Work out the finished part from the listing and answer in its coordinate system (mm). A direction names the side the tool comes from. Coordinates: 2 decimals unless noted, no trailing zeros. Order: outer loops, then holes, each group sorted by start corner. A loop starts at its lowest first (then second) coordinate and runs counter-clockwise, first axis right, second up.
1. The part is cut by section C-C, the plane z = 101.75. Give the vertices of the cut face in (x, y).
2. The part is cut by section A-A, the plane z = 10. Give the vertices of the cut face in (x, y), then the cut area to 4 significant figures.
3. The part is cut by section D-D, the plane x = 85. Give the vertices of the cut face in (y, z), then the cut area to 3 significant figures.
4. A tool of negligible diameter and unlimited length cuts with its end or side. For faces 1 (the flat face through (40, 15, 100)), 2 (the flat face through (8, 5, 16)), 3 (the flat face through (55, 10, 100)), from which of +Z, -Z, +X, -X, +Y, -Y can it reach the whole face along a straight path? Write none if from no direction.
5. The part is cut by section B-B, the plane x = 10. Give the vertices of the cut face in (y, z).
6. Find the intervals of material crossed by probe 1 along Z at (x, y) = (10, 12.75); probe 2 along Z at (x, y) = (85, 4); probe 3 along X at (y, z) = (10.5, 65), in increasing order.
7. Flat-ended cylindrical pins translate along their axes: pin 1 Ø5.5 at (x, z) = (58.25, 108.25) entering from -Y; pin 2 Ø3 at (x, z) = (20.61, 56.56) entering from +Y; pin 3 Ø3 at (y, z) = (11.5, 97) entering from -X; pin 4 Ø2 at (x, y) = (86.5, 7.5) entering from +Z. Find the tip coordinate at first contact, or state that the pin passes through.
8. Determine the mould class of faces 4 (the flat face through (0, 10, 41)), 5 (the cylindrical face through (37.54, 9.86, 5.38)), 6 (the flat face through (51, 0, 41)) for opening direction X: +X half, -X half, draft (parallel to the pull), parting line (faces both ways), or undercut.
Autodesk Inventor part; units mm, degrees
ref_plane "YZ Plane" through (0, 0, 0) normal (1, 0, 0) x (0, 1, 0)
ref_plane "XZ Plane" through (0, 0, 0) normal (0, 1, 0) x (-1, 0, 0)
ref_plane "XY Plane" through (0, 0, 0) normal (0, 0, 1) x (1, 0, 0)
sketch "Boceto1" plane through (0, 0, 0) normal (0, 1, 0) x (-1, 0, 0)
  line L0 (100, 80) -> (-100, 80)
  line L1 (-100, 80) -> (-100, -80)
  line L2 (-100, -80) -> (100, -80)
  line L3 (100, -80) -> (100, 80)
  line L4 (100, 80) -> (-100, -80) construction
  line L5 (-100, 80) -> (100, -80) construction
  point P0 (0, 0)
  dimension "d0" = 200
  dimension "d1" = 160
extrude "Extrusión1" add sketch "Boceto1" along normal blind 20
sketch "Boceto2" plane through (0, 20, 0) normal (0, 1, 0) x (1, 0, 0)
  line L0 (-100, 80) -> (-100, -80)
  line L1 (-100, 80) -> (-70, 80)
  line L2 (-70, 80) -> (-70, 40)
  line L3 (-70, 40) -> (-100, 40)
  line L4 (-100, 40) -> (-100, 80)
  line L5 (100, 80) -> (-100, 80)
  line L6 (0, 80) -> (0, 40)
  line L7 (100, 80) -> (70, 80)
  line L8 (70, 80) -> (70, 40)
  line L9 (70, 40) -> (100, 40)
  line L10 (100, 40) -> (100, 80)
  point P0 (0, 0)
  dimension "d4" = 30
  dimension "d5" = 40
extrude "Extrusión2" cut sketch "Boceto2" against normal blind 10
sketch "Boceto3" plane through (0, 20, 0) normal (0, 1, 0) x (1, 0, 0)
  line L0 (-70, 80) -> (-70, 40)
  line L1 (-70, 80.0001) -> (-70, 40)
  line L2 (-70, 40) -> (-100, 40)
  line L3 (-100, 40) -> (-100, 80.0001)
  line L4 (-100, 40) -> (-70, 40)
  line L5 (-70, 40) -> (-70, 80)
  line L6 (-70, 80) -> (-100, 80)
  line L7 (-100, 80) -> (-100, 40)
  circle A0 centre (-88.25, 58.25) radius 1.75
  circle A1 centre (-81.75, 51.75) radius 1.75
  line L8 (100, 80) -> (-100, 80)
  line L9 (0, 80) -> (0, 56.5)
  circle A2 centre (88.25, 58.25) radius 1.75
  circle A3 centre (81.75, 51.75) radius 1.75
  point P0 (0, 0)
  point P1 (-64.3507, 80)
  point P2 (-74.3507, 0)
  point P3 (-85, 80)
  dimension "d23" = 21.75
  dimension "d24" = 11.75
  dimension "d26" = 11.75
hole "Agujero1" at (-81.75, 20, -51.75) at (-88.25, 20, -58.25) at (81.75, 20, -51.75) at (88.25, 20, -58.25) direction (0, -1, 0) diameter 3.5 end through all
sketch "Boceto4" plane through (-100, 0, 80) normal (0, 0, 1) x (1, 0, 0)
  line L0 (30, 20) -> (60, 20)
  line L1 (60, 20) -> (60, 10)
  line L2 (60, 10) -> (30, 10)
  line L3 (30, 10) -> (30, 20)
  line L4 (0, 0) -> (0, 20)
  line L5 (100, 0) -> (100, 10)
  line L6 (170, 20) -> (140, 20)
  line L7 (140, 20) -> (140, 10)
  line L8 (140, 10) -> (170, 10)
  line L9 (170, 10) -> (170, 20)
  dimension "d34" = 30
  dimension "d35" = 10
  dimension "d36" = 30
extrude "Extrusión3" add sketch "Boceto4" along normal blind 40
sketch "Boceto5" plane through (0, 20, 0) normal (0, 1, 0) x (1, 0, 0)
  line L0 (59.9999, -50) -> (69.9999, -50)
  line L1 (49.9999, -101.75) -> (49.9999, -79.9497)
  line L2 (59.9999, -108.25) -> (59.9999, -50)
  line L3 (40, -80) -> (69.9999, -80)
  line L4 (49.9999, -79.9497) -> (40, -80)
  circle A0 centre (51.7499, -101.75) radius 1.75
  circle A1 centre (58.2499, -108.25) radius 1.75
  line L5 (69.9999, -80) -> (69.9999, -120)
  line L6 (40, -120) -> (40, -80)
  line L7 (69.9999, -120) -> (40, -120)
  line L8 (0, -50) -> (0, -71.75)
  line L9 (-40, -120) -> (-40, -80)
  line L10 (-49.9999, -101.75) -> (-49.9999, -79.9497)
  circle A2 centre (-51.7499, -101.75) radius 1.75
  circle A3 centre (-58.2499, -108.25) radius 1.75
  line L11 (-40, -80) -> (-69.9999, -80)
  line L12 (-69.9999, -120) -> (-40, -120)
  line L13 (-69.9999, -80) -> (-69.9999, -120)
  line L14 (-59.9999, -108.25) -> (-59.9999, -50)
  line L15 (-40, -120) -> (-69.9999, -120)
  line L16 (-69.9999, -80) -> (-69.9999, -120)
  line L17 (-40, -120) -> (-70, -120)
  line L18 (-40, -80) -> (-40, -120)
  line L19 (-59.9999, -110) -> (-49.9999, -110)
  line L20 (-49.9999, -110) -> (-49.9999, -100)
  line L21 (-49.9999, -100) -> (-59.9999, -100)
  line L22 (-59.9999, -100) -> (-59.9999, -110)
  line L23 (-100, 40) -> (-100, -80)
  point P0 (0, 0)
  point P1 (-56.75, -68.25)
  point P2 (-63.25, -61.75)
  point P3 (63.25, -61.75)
  point P4 (56.75, -68.25)
  dimension "d45" = 3.5
  dimension "d46" = 3.5
  dimension "d39" = 10
  dimension "d40" = 10
  dimension "d41" = 40
  dimension "d42" = 0
  dimension "d43" = 6.5
  dimension "d44" = 6.5
  dimension "d47" = 11.7499
  dimension "d48" = 11.75
  dimension "d49" = 0
  dimension "d50" = 11.75
  dimension "d51" = 0
  dimension "d97" = 40.0001
hole "Agujero2" at (-58.2499, 20, 108.25) at (-51.7499, 20, 101.75) at (51.7499, 20, 101.75) at (58.2499, 20, 108.25) direction (0, -1, 0) diameter 3.5 end through all
sketch "Boceto6" plane through (0, 20, 0) normal (0, 1, 0) x (1, 0, 0)
  circle A0 centre (-60.569, -13.1067) radius 10
  circle A1 centre (-29.569, -59.1067) radius 3.5
  line L0 (-60.569, -13.1067) -> (-39.0083, -13.1067)
  circle A2 centre (-29.569, 25.8933) radius 3.5
  circle A3 centre (-88.569, 25.8933) radius 3.5
  circle A4 centre (-88.569, -59.1067) radius 3.5
  line L1 (70.4544, -63.0517) -> (18.4544, -63.0517)
  line L2 (18.4544, -63.0517) -> (18.4544, 6.9483)
  line L3 (18.4544, 6.9483) -> (70.4544, 6.9483)
  line L4 (70.4544, 6.9483) -> (70.4544, -63.0517)
  line L5 (70.4544, 6.9483) -> (48.4544, 6.9483)
  line L6 (48.4544, 6.9483) -> (48.4544, 48.9483)
  line L7 (48.4544, 48.9483) -> (70.4544, 48.9483)
  line L8 (70.4544, 48.9483) -> (70.4544, 6.9483)
  line L9 (77.2288, -8.158) -> (77.2281, -5.6604)
  circle A5 centre (63.7706, -5.7606) radius 1.75
  line L10 (70.7641, -24.1464) -> (70.7641, 22.2796)
  circle A6 centre (35.8307, -5.7609) radius 1.75
  line L11 (25.1581, -13.2381) -> (25.1581, -10.7404)
  circle A7 centre (68.8507, -57.8309) radius 1.75
  line L12 (26.4277, 35.0051) -> (26.4277, 37.5029)
  circle A8 centre (20.6074, -56.5614) radius 1.75
  line L13 (18.6941, -55.9176) -> (70.7641, -55.9176)
  line L14 (18.6941, -55.9176) -> (18.6941, -7.6743)
  line L15 (44.7291, -55.9176) -> (44.7291, -31.7959)
  line L16 (63.7706, -28.0517) -> (26.4277, -28.0517)
  line L17 (44.7291, -23.5247) -> (44.7291, -31.7959)
  point P0 (0, 0)
  point P1 (-60.569, -16.6067)
  point P2 (45.425, 12.8886)
  point P3 (44.7291, -28.0517)
  dimension "d59" = 7
  dimension "d60" = 7
  dimension "d61" = 7
  dimension "d62" = 39
  dimension "d63" = 46
  dimension "d64" = 59
  dimension "d65" = 46
  dimension "d66" = 39
  dimension "d67" = 59
  dimension "d68" = 52
  dimension "d69" = 70
  dimension "d70" = 22
  dimension "d71" = 42
  dimension "d72" = 3.5
  dimension "d73" = 3.5
  dimension "d74" = 3.5
  dimension "d75" = 3.5
  dimension "d142" = 17.3763
  dimension "d143" = 12.7092
  dimension "d144" = 6.6837
  dimension "d145" = 12.7089
  dimension "d146" = 5.2208
  dimension "d147" = 1.6037
  dimension "d148" = 2.1531
  dimension "d149" = 6.4903
hole "Agujero3" at (68.8507, 20, 57.8309) at (20.6074, 20, 56.5614) at (63.7706, 20, 5.7606) at (35.8307, 20, 5.7609) direction (0, -1, 0) diameter 3.5 end through all
sketch "Boceto7" plane through (0, 20, 0) normal (0, 1, 0) x (1, 0, 0)
  circle A0 centre (-60.569, -13.1067) radius 10
  circle A1 centre (-29.569, -59.1067) radius 3.5
  line L0 (-60.569, -13.1067) -> (-39.0083, -13.1067)
  circle A2 centre (-29.569, 25.8933) radius 3.5
  circle A3 centre (-88.569, 25.8933) radius 3.5
  circle A4 centre (-88.569, -59.1067) radius 3.5
  point P0 (0, 0)
  point P1 (-60.569, -16.6067)
  dimension "d83" = 7
  dimension "d84" = 7
  dimension "d85" = 7
  dimension "d86" = 39
  dimension "d87" = 46
  dimension "d88" = 59
  dimension "d89" = 46
  dimension "d90" = 39
  dimension "d91" = 59
extrude "Extrusión4" cut sketch "Boceto7" against normal blind 20
ref_plane "Plano de trabajo1" through (0, 0, -80) normal (-1, 0, 0) x (0, 0, 1)
ref_plane "Plano de trabajo2" through (100, 0, 0) normal (0, 0, -1) x (-1, 0, 0)
sketch "Boceto8" plane through (0, 20, 0) normal (0, 1, 0) x (1, 0, 0)
  line L0 (80, -15) -> (90, -15)
  circle A0 centre (85, -10) radius 1.75
  line L1 (85, 10) -> (85, -10)
  line L2 (90, -15) -> (90, 15)
  circle A1 centre (85, 10) radius 1.75
  line L3 (80, 15) -> (80, -15)
  line L4 (90, 15) -> (80, -15) construction
  line L5 (80, 15) -> (90, -15) construction
  line L6 (90, 15) -> (80, 15)
  line L7 (100, -80) -> (100, 40)
  line L8 (0, 0) -> (20, -20)
  line L9 (0, 0) -> (28.2843, 0) construction
  line L10 (15, -60) -> (15, -70)
  circle A2 centre (10, -65) radius 1.75
  line L11 (-10, -65) -> (10, -65)
  line L12 (15, -70) -> (-15, -70)
  circle A3 centre (-10, -65) radius 1.75
  line L13 (-15, -60) -> (15, -60)
  line L14 (-15, -70) -> (15, -60) construction
  line L15 (-15, -60) -> (15, -70) construction
  line L16 (-15, -70) -> (-15, -60)
  line L17 (0, 0) -> (18.6615, 18.6615)
  line L18 (0, 0) -> (26.3913, 0) construction
  line L19 (-15, 60) -> (-15, 70)
  circle A4 centre (-10, 65) radius 1.75
  line L20 (10, 65) -> (-10, 65)
  line L21 (-15, 70) -> (15, 70)
  circle A5 centre (10, 65) radius 1.75
  line L22 (15, 60) -> (-15, 60)
  line L23 (15, 70) -> (-15, 60) construction
  line L24 (15, 60) -> (-15, 70) construction
  line L25 (15, 70) -> (15, 60)
  line L26 (70, 80) -> (-70, 80)
  line L27 (-40, -80) -> (40, -80)
  point P0 (86.9608, 0)
  point P1 (86.9608, 0)
  point P2 (85, 15)
  point P3 (0, -69.1269)
  point P4 (0, -69.1269)
  point P5 (-15, -67.1661)
  point P6 (0, 69.7066)
  point P7 (0, 69.7066)
  point P8 (15, 67.7458)
  point P9 (-15, 65)
  point P10 (15, -65)
  dimension "d98" = 10
  dimension "d99" = 30
  dimension "d100" = 10
  dimension "d101" = 5
  dimension "d102" = 5
  dimension "d103" = 5
  dimension "d104" = 5
  dimension "d105" = 45
  dimension "d106" = 45
  dimension "d107" = 10
  dimension "d108" = 10
  dimension "d109" = 30
  dimension "d110" = 5
  dimension "d111" = 5
  dimension "d112" = 5
  dimension "d113" = 5
  dimension "d114" = 10
  dimension "d115" = 30
  dimension "d116" = 5
  dimension "d117" = 5
  dimension "d118" = 5
  dimension "d119" = 5
  dimension "d120" = 10
hole "Agujero4" at (-10, 20, -65) at (10, 20, -65) at (85, 20, -10) at (85, 20, 10) at (10, 20, 65) at (-10, 20, 65) direction (0, -1, 0) diameter 3.5 end through all
sketch "Boceto9" plane through (0, 20, 0) normal (0, 1, 0) x (1, 0, 0)
  circle A0 centre (10, -10) radius 1.75
  line L0 (6.803, 0) -> (14.6069, 0)
  line L1 (0, 0) -> (0, -4.8284)
  line L2 (0, 0) -> (20.0354, 0)
  circle A1 centre (10, 10) radius 1.75
  line L3 (0, 0) -> (0, 4.8284)
  circle A2 centre (-10, 10) radius 1.75
  circle A3 centre (-10, -10) radius 1.75
  dimension "d128" = 3.5
  dimension "d129" = 10
  dimension "d130" = 10
hole "Agujero5" at (-10, 20, 10) at (-10, 20, -10) at (10, 20, -10) at (10, 20, 10) direction (0, -1, 0) diameter 3.5 end through all
sketch "Boceto10" plane through (0, 0, 0) normal (0, -1, 0) x (1, 0, 0)
  line L0 (-16, 16) -> (16, 16)
  line L1 (16, 16) -> (16, -16)
  line L2 (16, -16) -> (-16, -16)
  line L3 (-16, -16) -> (-16, 16)
  line L4 (-16, 16) -> (16, -16) construction
  line L5 (16, 16) -> (-16, -16) construction
  point P0 (0, 0)
  point P1 (0, 0)
  dimension "d138" = 32
  dimension "d139" = 32
extrude "Extrusión5" cut sketch "Boceto10" against normal blind 10
split "Dividir1" plane through (100, 0, 0) removes the side toward (0, 0, -1)
split "Dividir2" plane through (0, 0, -80) removes the side toward (-1, 0, 0)
properties part number "base_mid_4"
Geometry says:
1. outline: (40, 10) - (50, 10) - (50, 20) - (40, 20) - close; (53.5, 10) - (70, 10) - (70, 20) - (53.5, 20) - close
2. outline: (0, 10) - (8.25, 10) - (8.25, 20) - (0, 20) - close; (11.75, 10) - (16, 10) - (16, 0) - (83.25, 0) - (83.25, 20) - (11.75, 20) - close; (86.75, 0) - (100, 0) - (100, 20) - (86.75, 20) - close
2. area: 1,735 mm2
3. outline: (0, 0) - (20, 0) - (20, 8.25) - (0, 8.25) - close; (0, 11.75) - (20, 11.75) - (20, 80) - (0, 80) - close
3. area: 1,530 mm2
4. face 1: +Z, -X, +Y, -Y
4. face 2: -Z, -X, -Y
4. face 3: +Z, +X, -X, -Y
5. outline: (0, 16) - (10, 16) - (10, 11.75) - (20, 11.75) - (20, 63.25) - (0, 63.25) - close; (0, 66.75) - (20, 66.75) - (20, 80) - (0, 80) - close; (10, 0) - (20, 0) - (20, 8.25) - (10, 8.25) - close
6. probe 1: z = 0 to 8.25, 11.75 to 63.25, 66.75 to 80
6. probe 2: z = 0 to 8.25, 11.75 to 80
6. probe 3: x = 0 to 8.25, 11.75 to 100
7. pin 1: stops at y = 10
7. pin 2: passes through
7. pin 3: stops at x = 40
7. pin 4: stops at z = 80
8. face 4: -X half
8. face 5: undercut
8. face 6: draft
